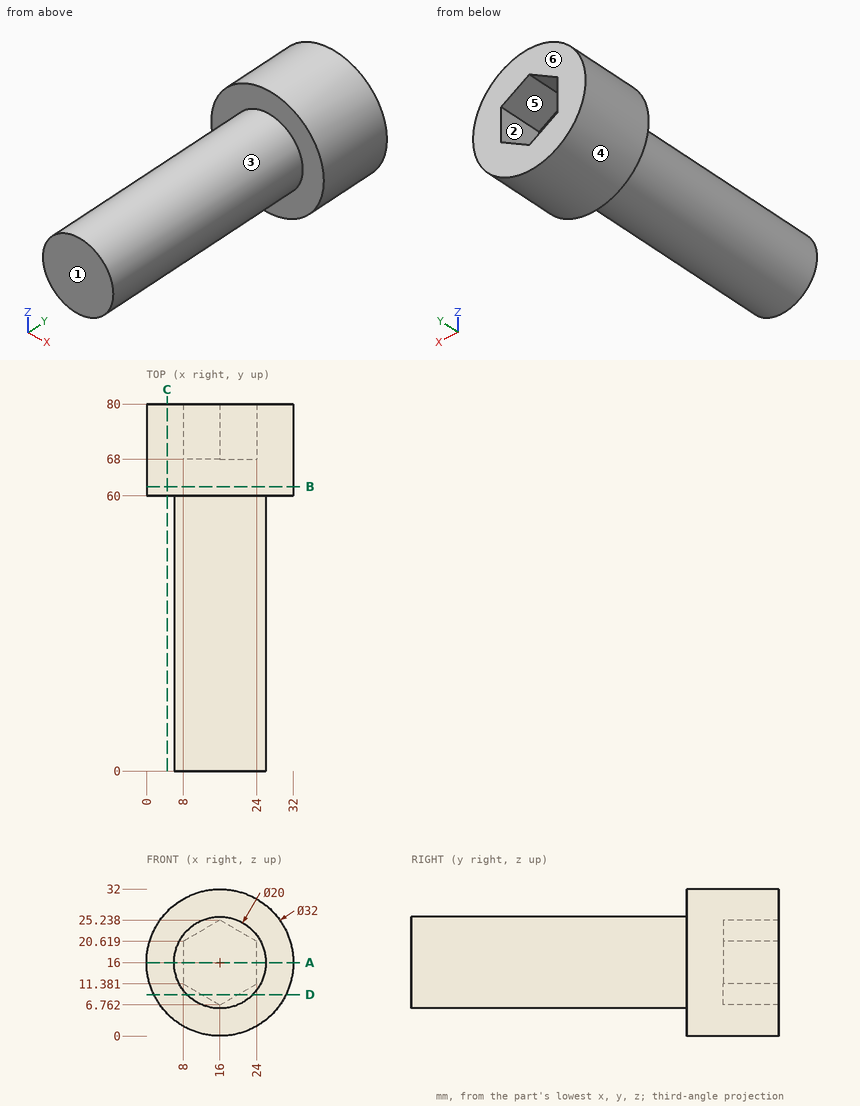
Drawing for the job (mm, zero at the part's lowest x, y, z). A direction names the side the tool comes from. Coordinates: 2 decimals unless noted, no trailing zeros. Order: outer loops, then holes, each group sorted by start corner. A loop starts at its lowest first (then second) coordinate and runs counter-clockwise, first axis right, second up. Notation, with made-up numbers: (66, 15) -> (96, 15) arc R15 ccw to (96, 24) -> close; hole circle Ø10 at (46.5, -24). An arc over 180 degrees is marked (long way). Answer in a Markdown table with one row per item.
1) Band-saw the part on A-A (z = 16). List the corners of the cut face in (x, y).
Check values:
| item | result |
|---|---|
| outline | (0, 60) -> (6, 60) -> (6, 0) -> (26, 0) -> (26, 60) -> (32, 60) -> (32, 80) -> (24, 80) -> (24, 68) -> (8, 68) -> (8, 80) -> (0, 80) -> close |
2) Which spindle directions (+Z, -Z, +X, -X, +Y, -Y) get a long thin tool onto all of the face, cutting with end or side? Do the marked faces 1, 2 and 3. Say none if no direction does.
Check values:
| item | result |
|---|---|
| face 1 | +Z, -Z, +X, -X, -Y |
| face 2 | +Y |
| face 3 | -Y |
3) Band-saw the part on C-C (x = 4.5). List the corners of the cut face in (y, z) (1 decimal), and give its area (3 significant figures).
Check values:
| item | result |
|---|---|
| outline | (60, 4.9) -> (80, 4.9) -> (80, 27.1) -> (60, 27.1) -> close |
| area | 445 mm2 |
4) Mould opens along X. For the marked faces 4, 5 and 6 say: pulls with the +X half, pulls with the -X half, needs draft (parallel to the pull), parting line crosses it, or undercut.
Check values:
| item | result |
|---|---|
| face 4 | parting line crosses it |
| face 5 | undercut |
| face 6 | needs draft |
5) Drill centre lines: line 1 (Y direction, x = 18.5, z = 14); line 2 (Y direction, x = 23.5, z = 7.5); line 3 (Z direction, x = 22, y = 32). Where is each one in solid material? Low to high.
Check values:
| item | result |
|---|---|
| line 1 | 0 to 68 |
| line 2 | 60 to 80 |
| line 3 | 8 to 24 |
6) Flat gauge pins, fed straight in: P1, Ø3, axis at y = 50, z = 18.5, coming from the +X side; P2, Ø10, axis at y = 74.5, z = 14, coming from the +X side; P3, Ø3, axis at x = 26, y = 66, coming from the -Z side (1 decimal); P4, Ø3, axis at y = 54, z = 15.5, coming from the +X side. Where does each tip first touch, or does it go through?
Check values:
| item | result |
|---|---|
| P1 | x = 25.95 |
| P2 | x = 32 |
| P3 | z = 2.4 |
| P4 | x = 26 |
7) Band-saw the part on D-D (z = 9). List the corners of the cut face in (x, y) (1 decimal).
Check values:
| item | result |
|---|---|
| outline | (1.6, 60) -> (8.9, 60) -> (8.9, 0) -> (23.1, 0) -> (23.1, 60) -> (30.4, 60) -> (30.4, 80) -> (19.9, 80) -> (19.9, 68) -> (12.1, 68) -> (12.1, 80) -> (1.6, 80) -> close |
8) Band-saw the part on B-B (y = 62). List the corners of the cut face in (x, z), and give its area (3 significant figures).
Check values:
| item | result |
|---|---|
| outline | circle Ø32 at (16, 16) |
| area | 804 mm2 |
